For this review, take the finished solid that the model builds, in its own axes (mm). Face numbers are marked on the shaded views. Give positions to 0.01 mm unless a question says otherwise; leave off trailing zeros. Write each loop counter-clockwise with the first axis right and the second up, starting at its lowest first coordinate (ties: lowest second). Pieces come first, ordered by that corner, then holes.
Q1. We need section A-A (x = 11.5). Write out the cut boundary in (y, z), then the cut area to 3 significant figures.
Q2. We need section B-B (z = 3). Write out the cut boundary in (x, y).
Q3. Mouldability with a two-part tool opening along Y and no side actions: class the marked faces 1, 2 and 3 as released by +Y, released by -Y, zero draft, split by the parting line, or undercut.
Q4. Insertion check: P1, Ø1, axis at x = 3.5, z = 10, coming from the -Y side; P2, Ø0.6, axis at y = 3.5, z = -5.5, coming from the -X side; P3, Ø0.6, axis at y = 3.5, z = -2.5, coming from the +X side. Each pin has a flat end and moves straight along its axis. Give the tip position at first contact, or say it passes through.
Q5. We need section C-C (z = 9). Write out the cut boundary in (x, y), then the cut area to 3 significant figures.
Q6. We need section D-D (z = 12.5). Write out the cut boundary in (x, y), then the cut area to 3 significant figures.
Q7. For line 1 (Y direction, x = -12.5, z = -10); line 2 (Z direction, x = 5, y = 4.65); line 3 (Y direction, x = 5, z = 13), list the stretches that pass through material, from the lowest coordinate up.
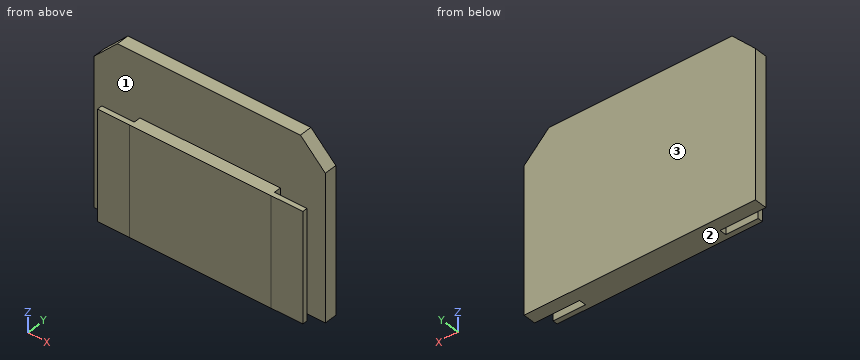
```python
from build123d import *

# Parameters (mm, degrees)
EXTRUDE_1_DEPTH          = 5.124133
EXTRUDE_1_DEPTH_BACK     = 12
EXTRUDE_2_DEPTH          = 10
CUT_EXTRUDE_1_DEPTH      = 25.003853471
CUT_EXTRUDE_1_DEPTH_BACK = 25.003853471


with BuildPart() as part:
    # 草图1 → 凸台-拉伸1 (new, two sides: drawn at the far end of the back side and taken through both)
    with BuildSketch(Plane.XY.offset(-EXTRUDE_1_DEPTH_BACK)):
        Polygon((-16.127330455, 4), (-16.127330455, 3.2), (-11.127330455, 3.2), (11.127330455, 3.200000056), (16.127758191, 3.200000069), (16.127758191, 4), (11.027330455, 4), (11.027330455, 5.1), (18.100330201, 5.1), (18.100330201, 7.1), (-18.227330455, 7.1), (-18.227330455, 5.1), (-11.027330455, 5.1), (-11.027330455, 4), align=None)
    extrude(amount=EXTRUDE_1_DEPTH + EXTRUDE_1_DEPTH_BACK)

    # 草图2 → 凸台-拉伸2 (add)
    with BuildSketch(Plane.XY.offset(5.12413323)):
        Polygon((11.027330455, 5.1), (-11.027330455, 5.1), (-18.227330455, 5.1), (-18.227330455, 7.1), (18.100330201, 7.1), (18.100330201, 5.1), align=None)
    extrude(amount=EXTRUDE_2_DEPTH)

    # 草图3 → 切除-拉伸1 (cut, two sides: drawn at the far end of the back side and taken through both)
    with BuildSketch(Plane(origin=(0, 7.1, 0), x_dir=(1, 0, 0), z_dir=(0, 1, 0)).offset(-CUT_EXTRUDE_1_DEPTH_BACK)):
        Polygon((18.100330201, -5.12413323), (18.100330201, -10.794403278), (18.100330201, -15.12413323), (-18.227330455, -15.12413323), (-18.227330455, -11.048403786), (-18.227330455, -5.12413323), (-20.378002423, -5.448805372), (-20.378002423, -17.361495583), (22.540888442, -17.361495583), (22.540888442, -5.12413323), align=None)
        Polygon((18.100330201, -15.12413323), (18.100330201, -10.794403278), (14.191406072, -14.703327407), (-14.572406834, -14.703327407), (-18.227330455, -11.048403786), (-18.227330455, -15.12413323), align=None)
    extrude(amount=CUT_EXTRUDE_1_DEPTH + CUT_EXTRUDE_1_DEPTH_BACK, mode=Mode.SUBTRACT)


solid = part.part
```
Computed:
1. outline: (3.2, -12) - (4, -12) - (4, 5.12) - (3.2, 5.12) - close; (5.1, -12) - (7.1, -12) - (7.1, 14.7) - (5.1, 14.7) - close
1. area: 67.1 mm2
2. outline: (-18.23, 5.1) - (-11.03, 5.1) - (-11.03, 4) - (-16.13, 4) - (-16.13, 3.2) - (16.13, 3.2) - (16.13, 4) - (11.03, 4) - (11.03, 5.1) - (18.1, 5.1) - (18.1, 7.1) - (-18.23, 7.1) - close
3. face 1: undercut
3. face 2: zero draft
3. face 3: released by +Y
4. P1: stops at y = 5.1
4. P2: stops at x = -16.13
4. P3: stops at x = 16.13
5. outline: (-18.23, 5.1) - (18.1, 5.1) - (18.1, 7.1) - (-18.23, 7.1) - close
5. area: 72.7 mm2
6. outline: (-16.78, 5.1) - (16.39, 5.1) - (16.39, 7.1) - (-16.78, 7.1) - close
6. area: 66.3 mm2
7. line 1: y = 3.2 to 4, 5.1 to 7.1
7. line 2: z = -12 to 5.12
7. line 3: y = 5.1 to 7.1
